Check sheet for the modelled part. Datum: model origin and axes. Units: mm. Round coordinates to 2 decimals unless told otherwise and drop trailing zeros. Loops run counter-clockwise (first coordinate to the right, second up) from the corner with the lowest first, then second, coordinate; pieces in that order, holes last. Notation, with made-up numbers: (81.25, 85.5) -> (137.25, 85.5) arc R30 ccw to (137.25, 124.5) -> close; hole circle Ø2 at (-16.5, 4). An arc over 180 degrees is marked (long way). Return JSON: item names as keys, results as strings.
from build123d import *

# Parameters (mm, degrees)
SKETCH1_W           = 46
SKETCH1_H           = 81
SKETCH1_R           = 1.25
BOSS_EXTRUDE1_DEPTH = 3
FILLET1_R           = 3
SKETCH4_R           = 1.9
CUT_EXTRUDE2_DEPTH  = 1.6
SKETCH5_R           = 1.65
CUT_EXTRUDE3_DEPTH  = 10


with BuildPart() as part:
    # Sketch1 → Boss-Extrude1 (new body)
    with BuildSketch(Plane.XY):
        Rectangle(SKETCH1_W, SKETCH1_H)
        with Locations((-20.3, 37.8)):
            Circle(SKETCH1_R, mode=Mode.SUBTRACT)
        with Locations(Location((20.3, 37.8, 0), (0, 0, 180))):
            Circle(SKETCH1_R, mode=Mode.SUBTRACT)
        with Locations((20.3, -37.8)):
            Circle(SKETCH1_R, mode=Mode.SUBTRACT)
        with Locations(Location((-20.3, -37.8, 0), (0, 0, 180))):
            Circle(SKETCH1_R, mode=Mode.SUBTRACT)
    extrude(amount=BOSS_EXTRUDE1_DEPTH)

    # Fillet1
    fillet1_edges = [part.edges().sort_by_distance(p)[0] for p in [
        (23, -40.5, 1.5),
        (-23, -40.5, 1.5),
        (-23, 40.5, 1.5),
        (23, 40.5, 1.5),
    ]]
    fillet(fillet1_edges, radius=FILLET1_R)

    # Sketch4 → Cut-Extrude2 (cut)
    with BuildSketch(Plane.XY.offset(3)):
        with Locations((20.3, 37.8)):
            Circle(SKETCH4_R)
        with Locations(Location((-20.3, 37.8, 0), (0, 0, 180))):
            Circle(SKETCH4_R)
        with Locations((-20.3, -37.8)):
            Circle(SKETCH4_R)
        with Locations(Location((20.3, -37.8, 0), (0, 0, 180))):
            Circle(SKETCH4_R)
    extrude(amount=-CUT_EXTRUDE2_DEPTH, mode=Mode.SUBTRACT)

    # Sketch5 → Cut-Extrude3 (cut)
    with BuildSketch(Plane.XY.offset(3)):
        with Locations((0, 30)):
            Circle(SKETCH5_R)
        with Locations(Location((0, -30, 0), (0, 0, 180))):
            Circle(SKETCH5_R)
    extrude(amount=-CUT_EXTRUDE3_DEPTH, mode=Mode.SUBTRACT)


solid = part.part
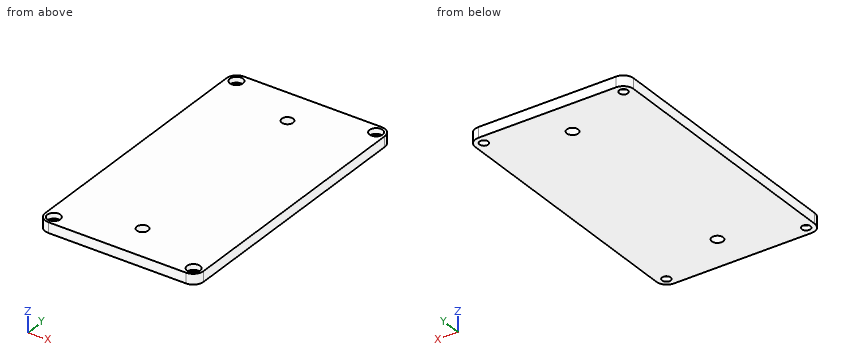
Q1. Section check B-B (z = 1.95). Record the boundary of the cut face in (x, y), then the cut area to 3 significant figures.
Results list:
{"outline": "(-23, -37.5) arc R3 ccw to (-20, -40.5) -> (20, -40.5) arc R3 ccw to (23, -37.5) -> (23, 37.5) arc R3 ccw to (20, 40.5) -> (-20, 40.5) arc R3 ccw to (-23, 37.5) -> close; hole circle Ø3.8 at (-20.3, -37.8); hole circle Ø3.8 at (-20.3, 37.8); hole circle Ø3.3 at (0, -30); hole circle Ø3.3 at (0, 30); hole circle Ø3.8 at (20.3, -37.8); hole circle Ø3.8 at (20.3, 37.8)", "area": "3,660 mm^2"}
Q2. Material ranges on line 1 (Y direction, x = 20.3, z = 0.7); line 2 (X direction, y = -37.8, z = 0.5); line 3 (Y direction, x = -20.3, z = 2.75), recorded low to high.
Results list:
{"line 1": "-40.48 to -39.05, -36.55 to 36.55, 39.05 to 40.48", "line 2": "-22.98 to -21.55, -19.05 to 19.05, 21.55 to 22.98", "line 3": "-40.48 to -39.7, -35.9 to 35.9, 39.7 to 40.48"}
Q3. Section check A-A (y = 30). Record the boundary of the cut face in (x, z), then the cut area to 3 significant figures.
Results list:
{"outline": "(-23, 0) -> (-1.65, 0) -> (-1.65, 3) -> (-23, 3) -> close; (1.65, 0) -> (23, 0) -> (23, 3) -> (1.65, 3) -> close", "area": "128 mm^2"}
Q4. Go/stop test with flat-tipped pins: pin 1 (1.9 mm diameter, centred on x = 21, y = 37.5, fed in from +Z); pin 2 (5 mm diameter, centred on x = -20.3, y = 37.8, fed in from +Z); pin 3 (2 mm diameter, centred on x = 0, y = -30, fed in from +Z). Record where each tip stops, or that it passes through.
Results list:
{"pin 1": "z = 1.4", "pin 2": "z = 3", "pin 3": "through"}
